The model under review builds one solid part; all positions refer to its coordinate system, in mm. A direction names the side the tool comes from. Round coordinates to 2 decimals unless told otherwise and drop trailing zeros. Order: outer loops, then holes, each group sorted by start corner. A loop starts at its lowest first (then second) coordinate and runs counter-clockwise, first axis right, second up. Notation, with made-up numbers: M -5,49.25 L 13,49.25 A19 cw 13,81.25 Z; hole C 85,80 d1. An arc over 180 degrees is marked long. Answer as a JSON object with one key per item and string values. Group by question number.
1) Consider section C-C, the plane z = 3. Write out the cut boundary in (x, y), then the cut area to 3 significant figures.
2) For faces 5 (the cylindrical face through (47.77, 4.29, 1.97)), 6 (the flat face through (12.3, 3.3, 4)), list the 3-axis set-ups (+Z, -Z, +X, -X, +Y, -Y) from which the entire face can be reached by the end or side of a thin tool; tool diameter is ignored.
3) The part is to be moulded in two halves that separate along Y. For faces 1 (the flat face through (0, 15, 4)), 2 (the cylindrical face through (13.417, 4.759, 5.972)), 3 (the flat face through (30, 30, 4)), 4 (the cylindrical face through (8.103, 2.79, 1.972)), say which applies: +Y half, -Y half, draft (parallel to the pull), parting line (faces both ways), or undercut.
4) Insertion check: pin 1 Ø7.5 at (x, y) = (51, 3.5) entering from +Z; pin 2 Ø5.5 at (x, y) = (50, 4) entering from +Z. Each pin has a flat end and moves straight along its axis. Give the tip position at first contact, or say it passes through.
5) Consider section D-D, the plane y = 20. Write out the cut boundary in (x, z).
6) Consider section B-B, the plane x = 50. Write out the cut boundary in (y, z).
7) To check wall thickness, follow line 1 (X direction, y = 20, z = 6.75); line 2 (X direction, y = 4.25, z = 6.25); line 3 (Y direction, x = 10, z = 1.95). State the ranges of each line that lie inside material, in increasing order.
8) Consider section A-A, the plane y = 4. Write out the cut boundary in (x, z).
Autodesk Inventor part; units mm, degrees
ref_plane "YZ Plane" through (0, 0, 0) normal (1, 0, 0) x (0, 1, 0)
ref_plane "XZ Plane" through (0, 0, 0) normal (0, 1, 0) x (-1, 0, 0)
ref_plane "XY Plane" through (0, 0, 0) normal (0, 0, 1) x (1, 0, 0)
sketch "Sketch1" plane through (0, 0, 0) normal (0, 0, 1) x (1, 0, 0)
  line L0 (0, 0) -> (60, 0)
  line L1 (60, 0) -> (60, 30)
  line L2 (60, 30) -> (0, 30)
  line L3 (0, 30) -> (0, 0)
  dimension "d0" = 60
  dimension "d1" = 30
extrude "Extrusion1" add sketch "Sketch1" along normal blind 8
sketch "Sketch2" plane through (0, 0, 8) normal (0, 0, 1) x (1, 0, 0)
  circle A0 centre (10, 4) radius 2
  circle A1 centre (50, 4) radius 2
  point P0 (0, 0)
hole "Hole1" at (10, 4, 8) at (50, 4, 8) direction (0, 0, -1) diameter 4.5 end through all counterbore diameter 7 counterbore depth 4
sketch "Sketch3" plane through (0, 0, 8) normal (0, 0, 1) x (1, 0, 0)
  line L0 (0, 0) -> (60, 0) construction
  line L1 (30, 0) -> (30, 50) construction
  line L2 (30, 0) -> (80, 0) construction
  line L3 (-6.3387, 20) -> (66.0929, 20) construction
  line L4 (0, 30) -> (0, 0)
  line L5 (60, 0) -> (60, 30)
  point P0 (50, 20)
  point P1 (10, 20)
  dimension "d11" = 50
  dimension "d12" = 90
  dimension "d13" = 20
  dimension "d14" = 10
  dimension "d15" = 10
hole "Hole2" at (50, 20, 8) at (10, 20, 8) direction (0, 0, -1) diameter 4.134 end through all
chamfer "Chamfer1" distance 0.1 angle 45 12 edges at (60, 15, 8) (30, 30, 8) (30, 0, 8) (0, 15, 8) (0, 15, 0) (30, 0, 0) (0, 0, 4) (60, 0, 4) (60, 15, 0) (60, 30, 4) (30, 30, 0) (0, 30, 4)
properties part number "Portal-Column-v2-Top" material "Aluminum 6061"
Results list:
{
 "1": {"outline": "M 0,0.1 L 0.1,0 L 59.9,0 L 60,0.1 L 60,29.9 L 59.9,30 L 0.1,30 L 0,29.9 Z; hole C 10,4 d4.5; hole C 10,20 d4.13; hole C 50,4 d4.5; hole C 50,20 d4.13", "area": "1,740 mm^2"},
 "2": {"face 5": "+Z, -Z", "face 6": "+Z"},
 "3": {"face 1": "draft", "face 2": "undercut", "face 3": "+Y half", "face 4": "undercut"},
 "4": {"pin 1": "z = 8", "pin 2": "z = 4"},
 "5": {"outline": "M 0,0.1 L 0.1,0 L 7.93,0 L 7.93,8 L 0.1,8 L 0,7.9 Z; M 12.07,0 L 47.93,0 L 47.93,8 L 12.07,8 Z; M 52.07,0 L 59.9,0 L 60,0.1 L 60,7.9 L 59.9,8 L 52.07,8 Z"},
 "6": {"outline": "M 0,0.1 L 0.1,0 L 1.75,0 L 1.75,4 L 0.5,4 L 0.5,8 L 0.1,8 L 0,7.9 Z; M 6.25,0 L 17.93,0 L 17.93,8 L 7.5,8 L 7.5,4 L 6.25,4 Z; M 22.07,0 L 29.9,0 L 30,0.1 L 30,7.9 L 29.9,8 L 22.07,8 Z"},
 "7": {"line 1": "0 to 7.93, 12.07 to 47.93, 52.07 to 60", "line 2": "0 to 6.51, 13.49 to 46.51, 53.49 to 60", "line 3": "0 to 1.75, 6.25 to 17.93, 22.07 to 30"},
 "8": {"outline": "M 0,0.1 L 0.1,0 L 7.75,0 L 7.75,4 L 6.5,4 L 6.5,8 L 0.1,8 L 0,7.9 Z; M 12.25,0 L 47.75,0 L 47.75,4 L 46.5,4 L 46.5,8 L 13.5,8 L 13.5,4 L 12.25,4 Z; M 52.25,0 L 59.9,0 L 60,0.1 L 60,7.9 L 59.9,8 L 53.5,8 L 53.5,4 L 52.25,4 Z"}
}
